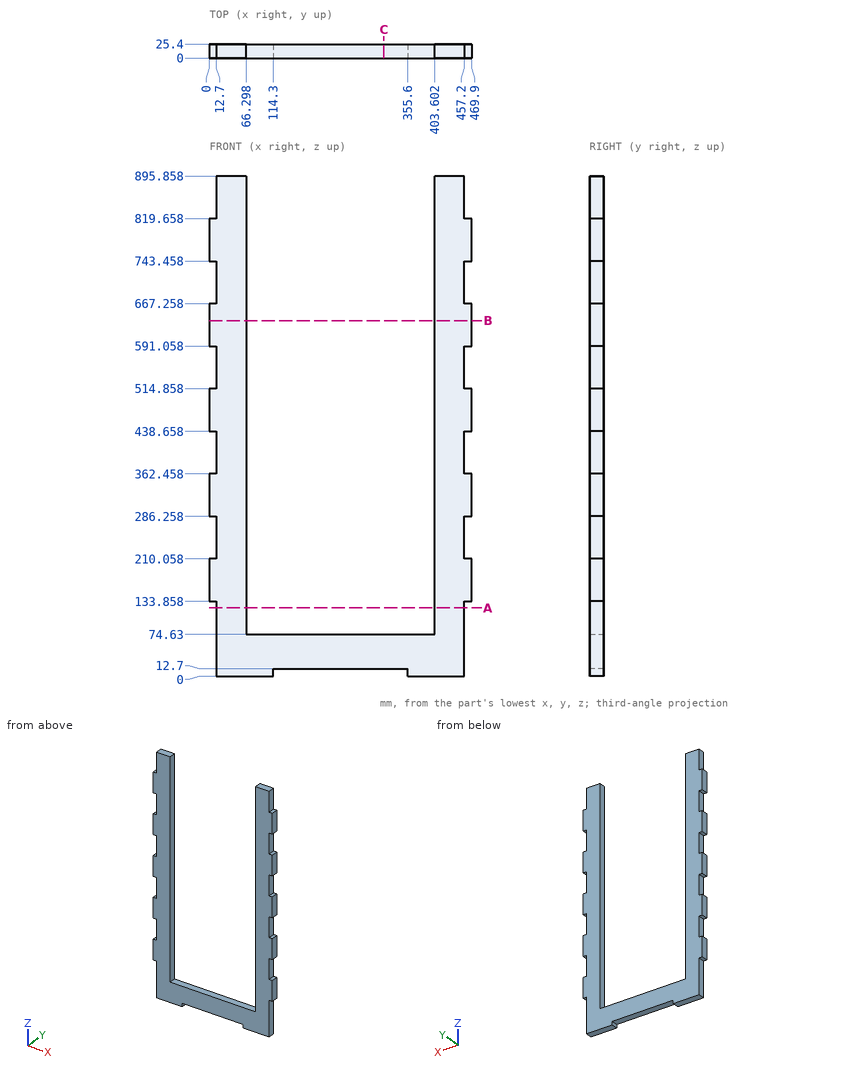
Geometry check sheet. Reference: drawing and pictorial views, mm from the part's lowest x, y, z. Round coordinates to 2 decimals unless told otherwise and drop trailing zeros. Loops run counter-clockwise (first coordinate to the right, second up) from the corner with the lowest first, then second, coordinate; pieces in that order, holes last. Notation, with made-up numbers: (84.25, 58) - (108.25, 58) arc R13 ccw to (108.25, 73) - close; hole circle Ø10 at (79, -4). An arc over 180 degrees is marked (long way). Write item = value, one per line. Start each with the question number.
Q1. Section check A-A (z = 122). Record the boundary of the cut face in (x, y).
Q2. Section check B-B (z = 637). Record the boundary of the cut face in (x, y).
Q3. Section check C-C (x = 313). Record the boundary of the cut face in (y, z).
Q4. Thickness scan on L1, parallel to X at y = 14, z = 132.5; L2, parallel to X at y = 20.75, z = 657.5; L3, parallel to Z at x = 180.5, y = 10.75. Record the ranges inside material, lowest first.
Q5. Depth check by flat-ended pin: P1, Ø10, axis at x = 464.5, y = 9.5, coming from the +Z side; P2, Ø12, axis at y = 16, z = 703, coming from the -X side; P3, Ø8, axis at x = 135, y = 8.5, coming from the +Z side. Enter the tip coordinate at first touch or a pass-through.
Derived:
q1.outline = (12.7, 0) - (66.3, 0) - (66.3, 25.4) - (12.7, 25.4) - close; (403.6, 0) - (457.2, 0) - (457.2, 25.4) - (403.6, 25.4) - close
q2.outline = (0, 0) - (66.3, 0) - (66.3, 25.4) - (0, 25.4) - close; (403.6, 0) - (469.9, 0) - (469.9, 25.4) - (403.6, 25.4) - close
q3.outline = (0, 12.7) - (25.4, 12.7) - (25.4, 74.63) - (0, 74.63) - close
q4.L1 = 12.7 to 66.3, 403.6 to 457.2
q4.L2 = 0 to 66.3, 403.6 to 469.9
q4.L3 = 12.7 to 74.63
q5.P1 = 819.66
q5.P2 = 12.7
q5.P3 = 74.63
